Design review of the part built by this model. Coordinates are the model's own, in mm. A direction names the side the tool comes from. Coordinates: 2 decimals unless noted, no trailing zeros. Write each loop counter-clockwise with the first axis right and the second up, starting at its lowest first coordinate (ties: lowest second). Pieces come first, ordered by that corner, then holes. Notation, with made-up numbers: M 13.5,50 L 41.5,50 A27 ccw 41.5,85 Z; hole C -13,17.5 d11. An arc over 180 degrees is marked long. One line per question, with ' | ' between items.
from build123d import *

# Parameters (mm, degrees)
SKETCH_R        = 6
PAD_DEPTH       = 10
PAD001_DEPTH    = 15
SKETCH002_R     = 2.2
POCKET_DEPTH    = 25.001
PAD002_DEPTH    = 3
SKETCH004_R     = 8.5
SKETCH004_R_2   = 4.25
PAD003_DEPTH    = 2
CHAMFER_SIZE    = 0.5
CHAMFER001_SIZE = 1


with BuildPart() as part:
    # Sketch → Pad (new body)
    with BuildSketch(Plane.XY):
        Circle(SKETCH_R)
    extrude(amount=PAD_DEPTH)

    # Sketch001 (on Face3 of Pad) → Pad001 (join)
    with BuildSketch(Plane.XY.offset(10)):
        with BuildLine():
            ThreePointArc((-3.6, -2.258871), (0, -4.25), (3.6, -2.258871))
            Line((3.6, -2.258871), (3.6, 2.258871))
            ThreePointArc((3.6, 2.258871), (0, 4.25), (-3.6, 2.258871))
            Line((-3.6, -2.258871), (-3.6, 2.258871))
        make_face()
    extrude(amount=PAD001_DEPTH)

    # Sketch002 (on Face8 of Pad001) → Pocket (cut, through all)
    with BuildSketch(Plane.XY.offset(25)):
        Circle(SKETCH002_R)
    extrude(amount=-POCKET_DEPTH, mode=Mode.SUBTRACT)

    # Sketch003 (on Face3 of Pocket) → Pad002 (join)
    with BuildSketch(Plane.XY.offset(10)):
        with BuildLine():
            ThreePointArc((3.776242, -1.95), (4.25, 0), (3.776242, 1.95))
            Line((3.776242, 1.95), (5.674284, 1.95))
            ThreePointArc((5.674284, -1.95), (6, 0), (5.674284, 1.95))
            Line((3.776242, -1.95), (5.674284, -1.95))
        make_face()
        with BuildLine():
            ThreePointArc((-1.148393, 5.889074), (-3, 5.196152), (-4.525892, 3.939074))
            Line((-3.57687, 2.295321), (-4.525892, 3.939074))
            ThreePointArc((-0.199371, 4.245321), (-2.125, 3.680608), (-3.57687, 2.295321))
            Line((-1.148393, 5.889074), (-0.199371, 4.245321))
        make_face()
        with BuildLine():
            ThreePointArc((-4.525892, -3.939074), (-3, -5.196152), (-1.148393, -5.889074))
            Line((-1.148393, -5.889074), (-0.199371, -4.245321))
            ThreePointArc((-3.57687, -2.295321), (-2.125, -3.680608), (-0.199371, -4.245321))
            Line((-4.525892, -3.939074), (-3.57687, -2.295321))
        make_face()
    extrude(amount=PAD002_DEPTH)

    # Sketch004 (on Face4 of Pad002) → Pad003 (join)
    with BuildSketch(Plane.XY.offset(10)):
        Circle(SKETCH004_R)
        Circle(SKETCH004_R_2, mode=Mode.SUBTRACT)
    extrude(amount=PAD003_DEPTH)

    # Chamfer
    chamfer_edges = [part.edges().sort_by_distance(p)[0] for p in [
        (-3.6, 0, 25),
        (0, 4.25, 25),
        (3.6, 0, 25),
        (0, -4.25, 25),
    ]]
    chamfer(chamfer_edges, length=CHAMFER_SIZE)

    # Chamfer001
    chamfer001_edges = [part.edges().sort_by_distance(p)[0] for p in [
        (-6, 0, 0),
    ]]
    chamfer(chamfer001_edges, length=CHAMFER001_SIZE)


solid = part.part
1. Insertion check: pin 1 Ø1 at (x, y) = (5, -4) entering from +Z; pin 2 Ø5 at (x, z) = (3.5, 15) entering from +Y; pin 3 Ø1.4 at (y, z) = (-0.5, 15) entering from +X. Each pin has a flat end and moves straight along its axis. Give the tip position at first contact, or say it passes through.
Answer sheet:
pin 1: z = 12 | pin 2: y = 4.13 | pin 3: x = 3.6
2. To check wall thickness, follow line 1 along Y through (x, z) = (0, 8.5); line 2 along Y through (x, z) = (0, 16.5); line 3 along X through (y, z) = (2, 13.25). State the ranges of each line that lie inside material, in increasing order. Write a range as [from, to].
Answer sheet:
line 1: [-6, -2.2], [2.2, 6] | line 2: [-4.25, -2.2], [2.2, 4.25] | line 3: [-3.6, -0.92], [0.92, 3.6]
3. Take a section at B-B (z = 23). Write out the cut boundary in (x, y).
Answer sheet:
outline: M -3.6,-2.26 A4.25 ccw 3.6,-2.26 L 3.6,2.26 A4.25 ccw -3.6,2.26 Z; hole C 0,0 d4.4
4. Take a section at A-A (y = 0). Write out the cut boundary in (x, z), then the cut area to 4 significant figures.
Answer sheet:
outline: M -8.5,10 L -6,10 L -6,1 L -5,0 L -2.2,0 L -2.2,25 L -3.1,25 L -3.6,24.5 L -3.6,10 L -4.25,10 L -4.25,12 L -8.5,12 Z; M 2.2,0 L 5,0 L 6,1 L 6,10 L 8.5,10 L 8.5,12 L 6,12 L 6,13 L 4.25,13 L 4.25,10 L 3.6,10 L 3.6,24.5 L 3.1,25 L 2.2,25 Z | area: 135.5 mm^2
5. Take a section at C-C (x = -6.75). Write out the cut boundary in (y, z), then the cut area to 3 significant figures.
Answer sheet:
outline: M -5.17,10 L 5.17,10 L 5.17,12 L -5.17,12 Z | area: 20.7 mm^2
6. Tool access review of faces 1 (the face through (-2.976, 5.21, 12.493)), 2 (the face through (2, 6, 10)), 3 (the face through (0.06, 4.25, 18.16)), 4 (the face through (-4.045, 3.106, 12.493)): name each direction out of +Z, -Z, +X, -X, +Y, -Y from which nothing blocks a thin tool from reaching the whole face with its end or side.
Answer sheet:
face 1: +Z, -X, +Y | face 2: -Z | face 3: +Z, +Y | face 4: +Z, -X
7. Draft analysis for pull direction Y (two halves, no side actions). For faces 5 (the face through (2.2, -1, 0)), 6 (the face through (-4.25, 0.03, 10.99)), 7 (the face through (4.57, 7.167, 10.986)), state which applies: pulls with the +Y half, pulls with the -Y half, needs draft (parallel to the pull), parting line crosses it, or undercut.
Answer sheet:
face 5: needs draft | face 6: undercut | face 7: parting line crosses it
